CAD build for the part. Positions are in the model's coordinates, mm. A direction names the side the tool comes from. Coordinates: 2 decimals unless noted, no trailing zeros. Loops run counter-clockwise (first coordinate to the right, second up) from the corner with the lowest first, then second, coordinate; pieces in that order, holes last. Notation, with made-up numbers: (78, 76) -> (130, 76) arc R11 cw to (130, 93) -> close; hole circle Ø7 at (80.5, 49). An arc over 180 degrees is marked (long way). Write item = value, one per line. Start each with the question number.
(1) Flat gauge pins, fed straight in: P1, Ø8, axis at y = 33, z = 506, coming from the -X side; P2, Ø5.5, axis at x = 16.5, y = 28.5, coming from the -Z side; P3, Ø3, axis at y = 35.82, z = 479.41, coming from the -X side; P4, Ø5, axis at x = 12.5, y = 28.5, coming from the +Z side. Where does each tip first touch, or does it go through?
(2) Band-saw the part on B-B (x = 17.25). Write the cut outline in (y, z) (3 decimals).
(3) Band-saw the part on C-C (z = 483). Write the cut outline in (x, y), and give its area (3 significant figures).
(4) Drill centre lines: line 1 (X direction, y = 26, z = 499); line 2 (Z direction, x = 22, y = 29.5); line 3 (Y direction, x = 18.75, z = 506.5). Where is each one in solid material? Low to high. Write a range as from..to.
(5) Band-saw the part on A-A (y = 29). Write the cut outline in (x, z).
(6) Tool access for faces 1 (the face through (17.563, 24.965, 534.851)), 2 (the face through (17, 25.665, 510)), 3 (the face through (17, 28, 502.475)): list every direction of +Z, -Z, +X, -X, +Y, -Y with a clear straight run to the whole face (end or side of a thin tool).
(7) Pull direction X, two halves, no side cores. Call faces 4 (the face through (22.423, 29.419, 484.167)), 5 (the face through (9.958, 29, 500)), 6 (the face through (19.958, 31, 489)): +X half, -X half, draft (parallel to the pull), parting line (faces both ways), or undercut.
(8) Band-saw the part on D-D (y = 25). Count the separate pieces of the cut face and the enclosed holes in it, and give its area (3 significant figures).
```python
from build123d import *

# Parameters (mm, degrees)
BOSS_EXTRUDE1_DEPTH = 2.54
BOSS_EXTRUDE2_DEPTH = 8.08
BOSS_EXTRUDE3_DEPTH = 5
BOSS_EXTRUDE4_START = 5
BOSS_EXTRUDE4_DEPTH = 5
SKETCH8_R           = 1.7
CUT_EXTRUDE1_DEPTH  = 16.0000001


with BuildPart() as part:
    # Sketch1 → Boss-Extrude1 (new body)
    with BuildSketch(Plane(origin=(14.957777778, 0, 0), x_dir=(0, 0, -1), z_dir=(1, 0, 0))):
        with BuildLine():
            Line((-496.113012561, 30.744895578), (-521.513012561, 30.744895578))
            Line((-521.513012561, 30.744895578), (-521.513012561, 25.664895578))
            Line((-521.513012561, 25.664895578), (-496.113012561, 25.664895578))
            ThreePointArc((-496.113012561, 25.664895578), (-494.404850963, 26.325059427), (-493.584615771, 27.962388527))
            Line((-493.584615771, 27.962388527), (-480.88314332, 33.756493956))
            ThreePointArc((-480.88314332, 33.756493956), (-477.098018282, 36.879077411), (-481.937324449, 36.067403333))
            Line((-481.937324449, 36.067403333), (-494.6387969, 30.273297904))
            ThreePointArc((-494.6387969, 30.273297904), (-495.339107499, 30.624124991), (-496.113012561, 30.744895578))
        make_face()
    extrude(amount=-BOSS_EXTRUDE1_DEPTH)

    # Sketch2 → Boss-Extrude2 (add)
    with BuildSketch(Plane(origin=(14.957777778, 0, 0), x_dir=(0, 0, -1), z_dir=(1, 0, 0))):
        with BuildLine():
            Line((-513.904615771, 25.664895578), (-502.474615771, 25.664895578))
            Line((-502.474615771, 25.664895578), (-502.474615771, 30.744895578))
            Line((-502.474615771, 30.744895578), (-530.414615771, 30.744895578))
            ThreePointArc((-530.414615771, 30.744895578), (-536.094228434, 29.404120904), (-540.574615771, 25.664895578))
            Line((-540.574615771, 25.664895578), (-540.574615771, 24.244992412))
            Line((-540.574615771, 24.244992412), (-539.304615771, 25.664895578))
            Line((-539.304615771, 25.664895578), (-538.034615771, 24.244992412))
            Line((-538.034615771, 24.244992412), (-536.764615771, 25.664895578))
            Line((-536.764615771, 25.664895578), (-535.494615771, 24.244992412))
            Line((-535.494615771, 24.244992412), (-534.224615771, 25.664895578))
            Line((-534.224615771, 25.664895578), (-532.954615771, 24.244992412))
            Line((-532.954615771, 24.244992412), (-531.684615771, 25.664895578))
            Line((-531.684615771, 25.664895578), (-530.414615771, 24.244992412))
            Line((-530.414615771, 24.244992412), (-529.144615771, 25.664895578))
            Line((-529.144615771, 25.664895578), (-527.874615771, 24.244992412))
            Line((-527.874615771, 24.244992412), (-526.604615771, 25.664895578))
            Line((-526.604615771, 25.664895578), (-525.334615771, 24.244992412))
            Line((-525.334615771, 24.244992412), (-524.064615771, 25.664895578))
            Line((-524.064615771, 25.664895578), (-522.794615771, 24.244992412))
            Line((-522.794615771, 24.244992412), (-521.524615771, 25.664895578))
            Line((-521.524615771, 25.664895578), (-520.254615771, 24.244992412))
            Line((-520.254615771, 24.244992412), (-518.984615771, 25.664895578))
            Line((-518.984615771, 25.664895578), (-517.714615771, 24.244992412))
            Line((-517.714615771, 24.244992412), (-516.444615771, 25.664895578))
            Line((-516.444615771, 25.664895578), (-515.174615771, 24.244992412))
            Line((-515.174615771, 24.244992412), (-513.904615771, 25.664895578))
        make_face()
    extrude(amount=BOSS_EXTRUDE2_DEPTH)

    # Sketch7 → Boss-Extrude3 (add)
    with BuildSketch(Plane(origin=(14.957777778, 0, 0), x_dir=(0, 0, -1), z_dir=(1, 0, 0))):
        with BuildLine():
            Line((-502.474615771, 30.744895578), (-479.408927659, 39.66518211))
            ThreePointArc((-479.408927659, 39.66518211), (-474.949798497, 37.8260107), (-476.562112461, 33.279932386))
            Line((-476.562112461, 33.279932386), (-491.562112461, 25.664895578))
            add(Edge.make_bspline(
                [(-491.562112461, 25.664895578), (-494.237137805, 24.306867814), (-495.170436648, 24.128959325), (-502.31030057, 22.103673482), (-507.062112461, 25.664895578), (-511.562112461, 25.664895578)],
                knots=[0, 0, 0, 0, 0.24107407, 0.34107407, 1, 1, 1, 1], degree=3))
            Line((-511.562112461, 25.664895578), (-513.904615771, 25.664895578))
            Line((-513.904615771, 25.664895578), (-515.174615771, 24.244992412))
            Line((-515.174615771, 24.244992412), (-516.444615771, 25.664895578))
            Line((-516.444615771, 25.664895578), (-517.714615771, 24.244992412))
            Line((-517.714615771, 24.244992412), (-518.984615771, 25.664895578))
            Line((-518.984615771, 25.664895578), (-520.254615771, 24.244992412))
            Line((-520.254615771, 24.244992412), (-521.524615771, 25.664895578))
            Line((-521.524615771, 25.664895578), (-522.794615771, 24.244992412))
            Line((-522.794615771, 24.244992412), (-524.064615771, 25.664895578))
            Line((-524.064615771, 25.664895578), (-525.334615771, 24.244992412))
            Line((-525.334615771, 24.244992412), (-526.604615771, 25.664895578))
            Line((-526.604615771, 25.664895578), (-527.874615771, 24.244992412))
            Line((-527.874615771, 24.244992412), (-529.144615771, 25.664895578))
            Line((-529.144615771, 25.664895578), (-530.414615771, 24.244992412))
            Line((-530.414615771, 24.244992412), (-531.684615771, 25.664895578))
            Line((-531.684615771, 25.664895578), (-532.954615771, 24.244992412))
            Line((-532.954615771, 24.244992412), (-534.224615771, 25.664895578))
            Line((-534.224615771, 25.664895578), (-535.494615771, 24.244992412))
            Line((-535.494615771, 24.244992412), (-536.764615771, 25.664895578))
            Line((-536.764615771, 25.664895578), (-538.034615771, 24.244992412))
            Line((-538.034615771, 24.244992412), (-539.304615771, 25.664895578))
            Line((-539.304615771, 25.664895578), (-540.574615771, 24.244992412))
            Line((-540.574615771, 24.244992412), (-540.574615771, 25.664895578))
            ThreePointArc((-540.574615771, 25.664895578), (-536.094228434, 29.404120904), (-530.414615771, 30.744895578))
            Line((-530.414615771, 30.744895578), (-502.474615771, 30.744895578))
        make_face()
    extrude(amount=-BOSS_EXTRUDE3_DEPTH)

    # Sketch7_2 → Boss-Extrude4 (add)
    with BuildSketch(Plane(origin=(14.957777778, 0, 0), x_dir=(0, 0, -1), z_dir=(1, 0, 0)).offset(BOSS_EXTRUDE4_START)):
        with BuildLine():
            Line((-502.474615771, 25.664895578), (-502.474615771, 30.744895578))
            Line((-502.474615771, 30.744895578), (-530.414615771, 30.744895578))
            ThreePointArc((-530.414615771, 30.744895578), (-536.094228434, 29.404120904), (-540.574615771, 25.664895578))
            Line((-540.574615771, 25.664895578), (-540.574615771, 24.244992412))
            Line((-540.574615771, 24.244992412), (-539.304615771, 25.664895578))
            Line((-539.304615771, 25.664895578), (-538.034615771, 24.244992412))
            Line((-538.034615771, 24.244992412), (-536.764615771, 25.664895578))
            Line((-536.764615771, 25.664895578), (-535.494615771, 24.244992412))
            Line((-535.494615771, 24.244992412), (-534.224615771, 25.664895578))
            Line((-534.224615771, 25.664895578), (-532.954615771, 24.244992412))
            Line((-532.954615771, 24.244992412), (-531.684615771, 25.664895578))
            Line((-531.684615771, 25.664895578), (-530.414615771, 24.244992412))
            Line((-530.414615771, 24.244992412), (-529.144615771, 25.664895578))
            Line((-529.144615771, 25.664895578), (-527.874615771, 24.244992412))
            Line((-527.874615771, 24.244992412), (-526.604615771, 25.664895578))
            Line((-526.604615771, 25.664895578), (-525.334615771, 24.244992412))
            Line((-525.334615771, 24.244992412), (-524.064615771, 25.664895578))
            Line((-524.064615771, 25.664895578), (-522.794615771, 24.244992412))
            Line((-522.794615771, 24.244992412), (-521.524615771, 25.664895578))
            Line((-521.524615771, 25.664895578), (-520.254615771, 24.244992412))
            Line((-520.254615771, 24.244992412), (-518.984615771, 25.664895578))
            Line((-518.984615771, 25.664895578), (-517.714615771, 24.244992412))
            Line((-517.714615771, 24.244992412), (-516.444615771, 25.664895578))
            Line((-516.444615771, 25.664895578), (-515.174615771, 24.244992412))
            Line((-515.174615771, 24.244992412), (-513.904615771, 25.664895578))
            Line((-513.904615771, 25.664895578), (-511.562112461, 25.664895578))
            Line((-511.562112461, 25.664895578), (-502.474615771, 25.664895578))
        make_face()
        with BuildLine():
            Line((-479.408927659, 39.66518211), (-502.474615771, 30.744895578))
            Line((-502.474615771, 30.744895578), (-502.474615771, 25.664895578))
            Line((-502.474615771, 25.664895578), (-511.562112461, 25.664895578))
            add(Edge.make_bspline(
                [(-491.562112461, 25.664895578), (-494.237137805, 24.306867814), (-495.170436648, 24.128959325), (-502.31030057, 22.103673482), (-507.062112461, 25.664895578), (-511.562112461, 25.664895578)],
                knots=[0, 0, 0, 0, 0.24107407, 0.34107407, 1, 1, 1, 1], degree=3))
            Line((-491.562112461, 25.664895578), (-476.562112461, 33.279932386))
            ThreePointArc((-476.562112461, 33.279932386), (-474.949798497, 37.8260107), (-479.408927659, 39.66518211))
        make_face()
    extrude(amount=BOSS_EXTRUDE4_DEPTH)

    # Sketch8 → Cut-Extrude1 (cut, through all)
    with BuildSketch(Plane(origin=(9.957777778, 0, 0), x_dir=(0, 0, -1), z_dir=(1, 0, 0))):
        with Locations((-496.113012561, 28.204895578)):
            Circle(SKETCH8_R)
        with Locations((-479.408927659, 35.824896282)):
            Circle(SKETCH8_R)
    extrude(amount=CUT_EXTRUDE1_DEPTH, mode=Mode.SUBTRACT)


solid = part.part
```
Findings below:
q1.P1 = 9.96
q1.P2 = 481.49
q1.P3 = through
q1.P4 = 540.31
q2.outline = (24.245, 515.175) -> (25.665, 513.905) -> (25.665, 502.475) -> (30.745, 502.475) -> (30.745, 530.415) arc R12.7 ccw to (25.665, 540.575) -> (24.245, 540.575) -> (25.665, 539.305) -> (24.245, 538.035) -> (25.665, 536.765) -> (24.245, 535.495) -> (25.665, 534.225) -> (24.245, 532.955) -> (25.665, 531.685) -> (24.245, 530.415) -> (25.665, 529.145) -> (24.245, 527.875) -> (25.665, 526.605) -> (24.245, 525.335) -> (25.665, 524.065) -> (24.245, 522.795) -> (25.665, 521.525) -> (24.245, 520.255) -> (25.665, 518.985) -> (24.245, 517.715) -> (25.665, 516.445) -> close
q3.outline = (9.96, 30.01) -> (14.96, 30.01) -> (14.96, 38.28) -> (9.96, 38.28) -> close; (19.96, 30.01) -> (24.96, 30.01) -> (24.96, 38.28) -> (19.96, 38.28) -> close
q3.area = 82.6 mm²
q4.line_1 = 9.96..14.96, 19.96..24.96
q4.line_2 = 484.01..495.01, 497.21..535.9
q4.line_3 = 25.66..30.74
q5.outline = (9.96, 484.99) -> (14.96, 484.99) -> (14.96, 494.61) -> (9.96, 494.61) -> close; (9.96, 497.62) -> (14.96, 497.62) -> (14.96, 502.47) -> (19.96, 502.47) -> (19.96, 497.62) -> (24.96, 497.62) -> (24.96, 536.84) -> (9.96, 536.84) -> close; (19.96, 484.99) -> (24.96, 484.99) -> (24.96, 494.61) -> (19.96, 494.61) -> close
q6.face_1 = +X, -X, -Y
q6.face_2 = -Y
q6.face_3 = -Z, +Y, -Y
q7.face_4 = draft
q7.face_5 = -X half
q7.face_6 = undercut
q8.separate_pieces = 13
q8.enclosed_holes = 0
q8.area = 359 mm²
